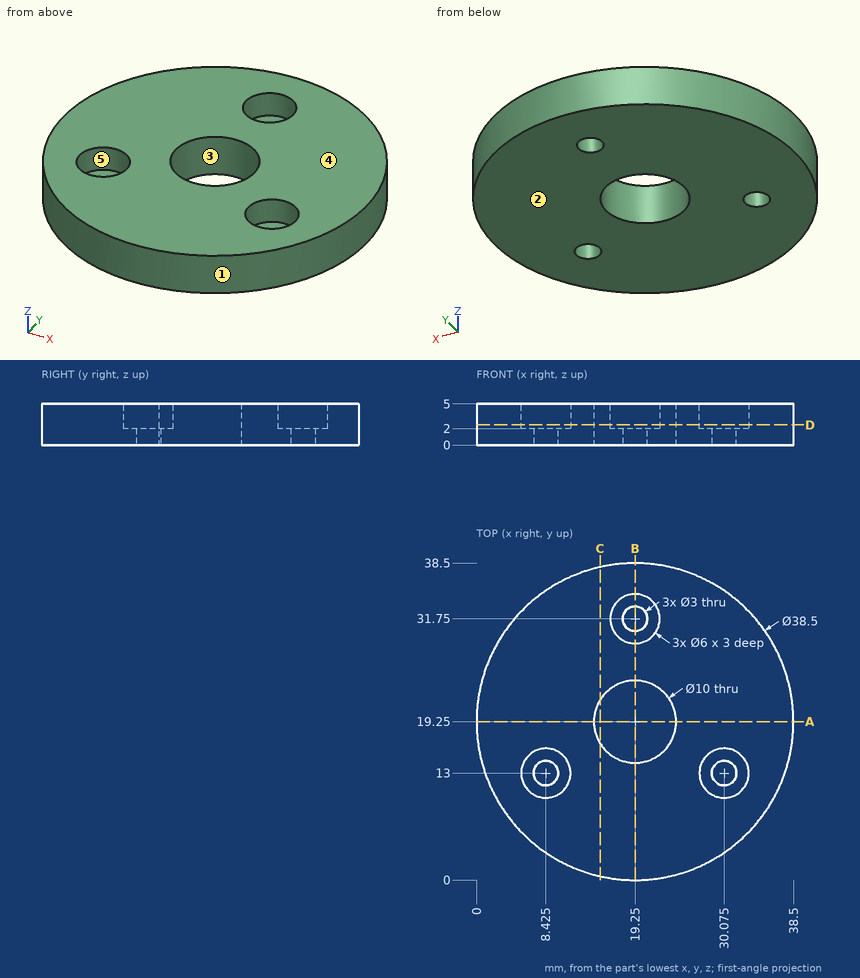
Job drawing, mm, ordinate dimensions from the low corner. One solid piece. A direction names the side the tool comes from. Coordinates: 2 decimals unless noted, no trailing zeros. Order: outer loops, then holes, each group sorted by start corner. A loop starts at its lowest first (then second) coordinate and runs counter-clockwise, first axis right, second up. Notation, with made-up numbers: (71.5, -37.75) -> (84.5, -37.75) arc R19 cw to (84.5, -27.75) -> close; hole circle Ø11 at (-19.75, 71). An arc over 180 degrees is marked (long way). Answer in a Markdown table with one row per item. Add a question column.
Q1. Band-saw the part on B-B, the plane x = 19.25. List the corners of the cut face in (y, z).
Q2. Band-saw the part on C-C, the plane x = 15. List the corners of the cut face in (y, z) (1 decimal).
Q3. Drop flat-ended pins along their axis: pin 1 (2 mm diameter, centred on x = 30.5, z = 3, fed in from +Y) (1 decimal); pin 2 (3 mm diameter, centred on x = 30, z = 1, fed in from +Y); pin 3 (1 mm diameter, centred on x = 19.5, z = 2.5, fed in from -Y); pin 4 (8 mm diameter, centred on x = 10.5, y = 20, fed in from -Z). Give the stop position or say it passes through.
Q4. Mould opens along Y. For the marked faces 1, 2 and 3 say: +Y half, -Y half, draft (parallel to the pull), parting line (faces both ways), or undercut.
Q5. Band-saw the part on A-A, the plane y = 19.25. List the corners of the cut face in (x, z), then the cut area to 4 significant figures.
Q6. Which spindle directions (+Z, -Z, +X, -X, +Y, -Y) get a long thin tool onto all of the face, cutting with end or side? Do the marked faces 4 and 5. Say none if no direction does.
Q7. Wall check: line 1 along Y through (x, z) = (19.25, 3.8); line 2 along X through (y, z) = (13, 0.75) (1 decimal); line 3 along X through (y, z) = (11, 3.95). Give the ranges that are in metal, low to high. Write a range as [from, to].
Q8. Band-saw the part on D-D, the plane z = 2.45. Give the number of separate pieces and of enclosed holes in the cut face, then the cut area to 3 significant figures.
Answers follow:
| question | item | result |
|---|---|---|
| 1 | outline | (0, 0) -> (14.25, 0) -> (14.25, 5) -> (0, 5) -> close; (24.25, 0) -> (30.25, 0) -> (30.25, 2) -> (28.75, 2) -> (28.75, 5) -> (24.25, 5) -> close; (33.25, 0) -> (38.5, 0) -> (38.5, 5) -> (34.75, 5) -> (34.75, 2) -> (33.25, 2) -> close |
| 2 | outline | (0.5, 0) -> (16.6, 0) -> (16.6, 5) -> (0.5, 5) -> close; (21.9, 0) -> (38, 0) -> (38, 5) -> (21.9, 5) -> close |
| 3 | pin 1 | y = 35.5 |
| 3 | pin 2 | y = 36.13 |
| 3 | pin 3 | y = 0 |
| 3 | pin 4 | z = 0 |
| 4 | face 1 | parting line |
| 4 | face 2 | draft |
| 4 | face 3 | undercut |
| 5 | outline | (0, 0) -> (14.25, 0) -> (14.25, 5) -> (0, 5) -> close; (24.25, 0) -> (38.5, 0) -> (38.5, 5) -> (24.25, 5) -> close |
| 5 | area | 142.5 mm^2 |
| 6 | face 4 | +Z, +X, -X, +Y, -Y |
| 6 | face 5 | +Z |
| 7 | line 1 | [0, 14.25], [24.25, 28.75], [34.75, 38.5] |
| 7 | line 2 | [1, 6.9], [9.9, 28.6], [31.6, 37.5] |
| 7 | line 3 | [1.86, 6.19], [10.66, 27.84], [32.31, 36.64] |
| 8 | separate pieces | 1 |
| 8 | enclosed holes | 4 |
| 8 | area | 1,000 mm^2 |
